Verification items for the finished model (mm, model axes). A direction names the side the tool comes from. Round coordinates to 2 decimals unless told otherwise and drop trailing zeros. Write each loop counter-clockwise with the first axis right and the second up, starting at its lowest first coordinate (ties: lowest second). Pieces come first, ordered by that corner, then holes. Notation, with made-up numbers: (31, -9.5) - (82, -9.5) arc R25 cw to (82, 6.5) - close; hole circle Ø7 at (22.25, 34). An arc over 180 degrees is marked (long way). Answer as a JSON object with one key per item and string values.
```python
from build123d import *

# Parameters (mm, degrees)
F1_DEPTH = 400
F2_W     = 1400
F2_H     = 250
F2_H_2   = 90
F3_DEPTH = 500.001
F4_W     = 1100
F4_H     = 200
F5_DEPTH = 400


with BuildPart() as f1:
    # F0 (on Top) → F1 (new body)
    with BuildSketch(Plane.XY):
        Polygon((1250, 0), (150, 0), (0, -150), (0, -350), (150, -500), (1250, -500), (1400, -350), (1400, -150), align=None)
    extrude(amount=F1_DEPTH)

    # F2 (on face) → F3 (cut, through all)
    with BuildSketch(Plane(origin=(0, 0, 0), x_dir=(-1, 0, 0), z_dir=(0, 1, 0))):
        with Locations((-700, 155)):
            Rectangle(F2_W, F2_H)
        with Locations((-700, 355)):
            Rectangle(F2_W, F2_H_2)
    extrude(amount=-F3_DEPTH, mode=Mode.SUBTRACT)

    # F4 (on face) → F5 (join)
    with BuildSketch(Plane(origin=(0, 0, 0), x_dir=(1, 0, 0), z_dir=(0, 0, -1))):
        with Locations((700, 250)):
            Rectangle(F4_W, F4_H)
    extrude(amount=-F5_DEPTH)


solid = f1.part
```
1. Mould release check, pull along Z, two halves, no side actions. Record for faces 1 (the face through (692, -500, 295)), 2 (the face through (692, -251, 400)), 3 (the face through (710, -358, 30)): released by +Z, released by -Z, zero draft, split by the parting line, or undercut.
Completed:
{"face 1": "zero draft", "face 2": "released by +Z", "face 3": "undercut"}
2. Cross-section at A-A (y = -75). Record the boundary of the cut face in (x, z).
Completed:
{"outline": "(75, 0) - (1325, 0) - (1325, 30) - (75, 30) - close; (75, 280) - (1325, 280) - (1325, 310) - (75, 310) - close"}
3. Cross-section at D-D (x = 650). Record the boundary of the cut face in (y, z), plus the area to 3 significant figures.
Completed:
{"outline": "(-500, 0) - (0, 0) - (0, 30) - (-150, 30) - (-150, 280) - (0, 280) - (0, 310) - (-150, 310) - (-150, 400) - (-350, 400) - (-350, 310) - (-500, 310) - (-500, 280) - (-350, 280) - (-350, 30) - (-500, 30) - close", "area": "98,000 mm^2"}
4. Cross-section at B-B (x = 1294). Record the boundary of the cut face in (y, z), plus the area to 3 significant figures.
Completed:
{"outline": "(-456, 0) - (-44, 0) - (-44, 30) - (-456, 30) - close; (-456, 280) - (-44, 280) - (-44, 310) - (-456, 310) - close", "area": "24,700 mm^2"}
5. Cross-section at C-C (y = -270). Record the boundary of the cut face in (x, z), plus the area to 3 significant figures.
Completed:
{"outline": "(0, 0) - (1400, 0) - (1400, 30) - (1250, 30) - (1250, 280) - (1400, 280) - (1400, 310) - (1250, 310) - (1250, 400) - (150, 400) - (150, 310) - (0, 310) - (0, 280) - (150, 280) - (150, 30) - (0, 30) - close", "area": "458,000 mm^2"}
6. Material ranges on probe 1 along Z at (x, y) = (768, -354); probe 2 along X at (y, z) = (-181.5, 358.5); probe 3 along Y at (x, z) = (189, 226.5), recorded low to high. Write a range as from..to.
Completed:
{"probe 1": "z = 0..30, 280..310", "probe 2": "x = 150..1250", "probe 3": "y = -350..-150"}
7. Access from +Z, -Z, +X, -X, +Y, -Y to the whole of each face (thin tool, end or side, straight path). Record for faces 4 (the face through (1250, -249, 153)), 5 (the face through (692, -350, 153)), 6 (the face through (0, -249, 295)), 7 (the face through (150, -249, 354)).
Completed:
{"face 4": "+X, +Y, -Y", "face 5": "+X, -X, -Y", "face 6": "+Z, -Z, -X, +Y, -Y", "face 7": "+Z, -X, +Y, -Y"}
8. Go/stop test with flat-tipped pins: pin 1 (5 mm diameter, centred on x = 186, z = 199, fed in from -Y); pin 2 (8 mm diameter, centred on x = 605.5, z = 157, fed in from +Y). Record where each tip stops, or that it passes through.
Completed:
{"pin 1": "stops at y = -350", "pin 2": "stops at y = -150"}
